```python
from build123d import *

# Parameters (mm, degrees)
CUT_EXTRUDE1_START = -16
SKETCH2_R          = 5
CUT_EXTRUDE1_DEPTH = 252
CIRPATTERN1_COUNT  = 8


with BuildPart() as part:
    # Sketch1 → Revolve1 (revolve)
    with BuildSketch(Plane.XY):
        Polygon((143.5, 250), (143.5, 0), (182.5, 0), (182.5, 15), (150, 15), (150, 250), align=None)
    revolve(axis=Axis((0, 0, 0), (0, 1, 0)))

    # Sketch2 → Cut-Extrude1 (cut)
    with BuildSketch(Plane(origin=(0, 15, 0), x_dir=(1, 0, 0), z_dir=(0, 1, 0)).offset(CUT_EXTRUDE1_START)):
        with Locations((159.369219358, 66.012892083)):
            Circle(SKETCH2_R)
    cut_extrude1 = extrude(amount=CUT_EXTRUDE1_DEPTH, mode=Mode.SUBTRACT)

    # CirPattern1: Cut-Extrude1 ×8 about axis
    cirpattern1_axis = Axis((0, 0, 0), (0, 1, 0))
    for i in range(1, CIRPATTERN1_COUNT):
        add(cut_extrude1.rotate(cirpattern1_axis, i * 360 / CIRPATTERN1_COUNT), mode=Mode.SUBTRACT)


solid = part.part
```
CAD build for the part. Positions are in the model's coordinates, mm. A direction names the side the tool comes from. Round coordinates to 2 decimals unless told otherwise and drop trailing zeros. Order: outer loops, then holes, each group sorted by start corner. A loop starts at its lowest first (then second) coordinate and runs counter-clockwise, first axis right, second up. Notation, with made-up numbers: (66, 47.5) - (105, 47.5) arc R11 ccw to (105, 55.5) - close; hole circle Ø9 at (57.25, 53). An arc over 180 degrees is marked (long way). Use CSV: the item, a comma, the result in double quotes. Start each with the question number.
1) Saw through at C-C (y = 227.5). List the corners of the cut face in (x, z).
2) Saw through at A-A (x = 0). List the corners of the cut face in (y, z), and give its area (4 significant figures).
3) Saw through at B-B (z = 0). List the corners of the cut face in (x, y).
4) Wall check: L1, parallel to Z at x = 0, y = 182; L2, parallel to X at y = 39, z = 115.5. Give the ranges that are in metal, low to high. Write a range as [from, to].
5) Two-plate mould, pull along Z, no slides. Class faces 1 (the cylindrical face through (-19.527, 134.145, -148.724)), 2 (the flat face through (122, 250, 77)), 3 (the cylindrical face through (136.873, 123.25, -43.104)): pulls with the +Z half, pulls with the -Z half, needs draft (parallel to the pull), parting line crosses it, or undercut.
6) Tool access for faces 4 (the cylindrical face through (-68.323, 7.395, 163.803)), 5 (the flat face through (13, 15, -150)): list every direction of +Z, -Z, +X, -X, +Y, -Y with a clear straight run to the whole face (end or side of a thin tool).
7) Pin check, flat tips, straight feed: pin 1 Ø3 at (x, y) = (17.5, 71.5) entering from +Z; pin 2 Ø6 at (x, z) = (159.37, 66.01) entering from +Y (3 decimals); pin 3 Ø4 at (y, z) = (189, 82) entering from +X; pin 4 Ø11.5 at (x, z) = (-159.37, 66.01) entering from +Y. Stop position of each tip, or through.
Values follow:
1,outline,"circle Ø300 at (0, 0); hole circle Ø287 at (0, 0)"
2,outline,"(0, -182.5) - (15, -182.5) - (15, -150) - (250, -150) - (250, -143.5) - (0, -143.5) - close; (0, 143.5) - (250, 143.5) - (250, 150) - (15, 150) - (15, 182.5) - (0, 182.5) - close"
2,area,"4,225 mm2"
3,outline,"(-182.5, 0) - (-143.5, 0) - (-143.5, 250) - (-150, 250) - (-150, 15) - (-182.5, 15) - close; (143.5, 0) - (182.5, 0) - (182.5, 15) - (150, 15) - (150, 250) - (143.5, 250) - close"
4,L1,"z = [-150, -143.5], [143.5, 150]"
4,L2,"x = [-95.71, -85.16], [85.16, 95.71]"
5,face 1,"parting line crosses it"
5,face 2,"needs draft"
5,face 3,"undercut"
6,face 4,"+Y, -Y"
6,face 5,"+Y"
7,pin 1,"stops at z = 149.14"
7,pin 2,"passes through"
7,pin 3,"stops at x = 126.89"
7,pin 4,"stops at y = 15"
